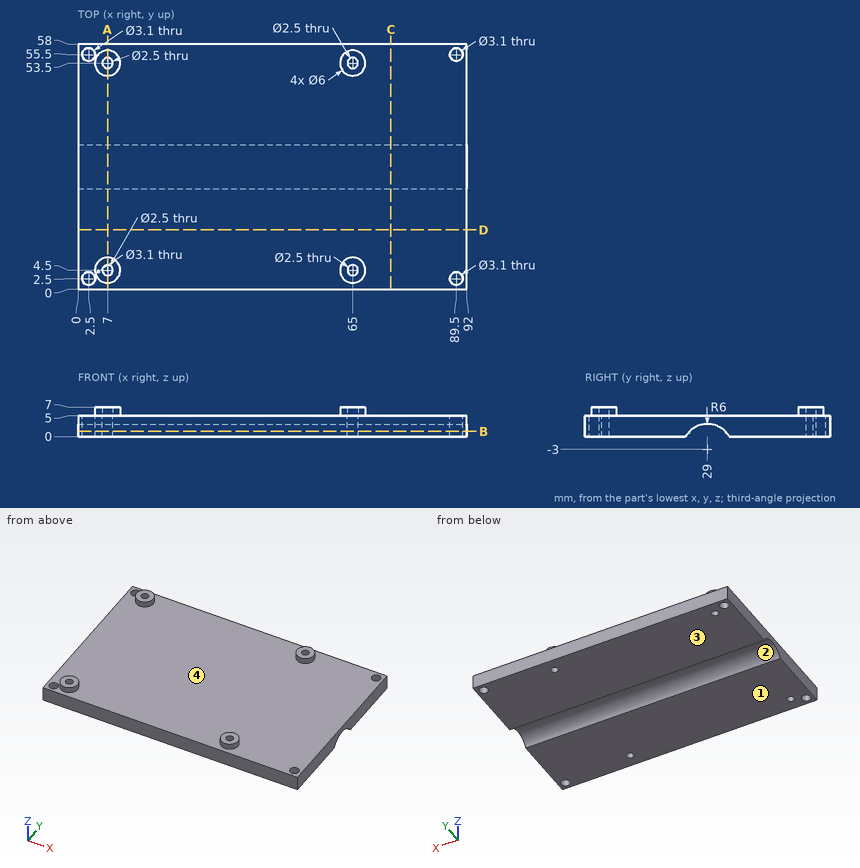
Check sheet for the drawn part. Datum: minimum x, y, z corner. Units: mm. A direction names the side the tool comes from. Round coordinates to 2 decimals unless told otherwise and drop trailing zeros. Order: outer loops, then holes, each group sorted by start corner. A loop starts at its lowest first (then second) coordinate and runs counter-clockwise, first axis right, second up.
(1) Go/stop test with flat-tipped pins: P1, Ø6, axis at x = 46, y = 19, coming from the +Z side; P2, Ø1.9, axis at x = 89.5, y = 55.5, coming from the +Z side. Record where each tip stops, or that it passes through.
(2) Draft check along Y on the marked faces 1 and 2. Enter one of: pulls with the +Y half, pulls with the -Y half, needs draft (parallel to the pull), parting line crosses it, or undercut.
(3) Cross-section at D-D, the plane y = 14. Enter the section's corners in (x, z).
(4) Access from +Z, -Z, +X, -X, +Y, -Y to the whole of each face (thin tool, end or side, straight path). Record for the marked faces 3 and 4.
(5) Cross-section at B-B, the plane z = 1.25. State how many separate pieces and enclosed holes the cut face has, and give its area (3 significant figures).
(6) Cross-section at C-C, the plane x = 74. Enter the section's corners in (y, z).
(7) Cross-section at A-A, the plane x = 7. Enter the section's corners in (y, z), and give its area (3 significant figures).
(8) Scan lines: probe 1 along X at (y, z) = (53.5, 2.25); probe 2 along Y at (x, z) = (65, 5.5); probe 3 along Y at (x, z) = (65, 4). Record each from-to range of solid material in increasing order.
Check sheet entries:
1. P1: stops at z = 5
1. P2: passes through
2. face 1: needs draft
2. face 2: undercut
3. outline: (0, 0) - (92, 0) - (92, 5) - (0, 5) - close
4. face 3: -Z, +X, -X, +Y, -Y
4. face 4: +Z
5. separate pieces: 2
5. enclosed holes: 8
5. area: 4,510 mm2
6. outline: (0, 0) - (23.8, 0) arc R6 cw to (34.2, 0) - (58, 0) - (58, 5) - (0, 5) - close
7. outline: (0, 0) - (3.25, 0) - (3.25, 7) - (1.5, 7) - (1.5, 5) - (0, 5) - close; (5.75, 0) - (23.8, 0) arc R6 cw to (34.2, 0) - (52.25, 0) - (52.25, 7) - (50.5, 7) - (50.5, 5) - (7.5, 5) - (7.5, 7) - (5.75, 7) - close; (54.75, 0) - (58, 0) - (58, 5) - (56.5, 5) - (56.5, 7) - (54.75, 7) - close
7. area: 257 mm2
8. probe 1: x = 0 to 5.75, 8.25 to 63.75, 66.25 to 92
8. probe 2: y = 1.5 to 3.25, 5.75 to 7.5, 50.5 to 52.25, 54.75 to 56.5
8. probe 3: y = 0 to 3.25, 5.75 to 52.25, 54.75 to 58
